Here's how the part is built. I have some questions about the finished solid (model axes, mm). A direction names the side the tool comes from. Round coordinates to 2 decimals unless told otherwise and drop trailing zeros. Loops run counter-clockwise (first coordinate to the right, second up) from the corner with the lowest first, then second, coordinate; pieces in that order, holes last. Notation, with made-up numbers: (75.25, -14.5) -> (128.25, -14.5) arc R14 ccw to (128.25, 10.5) -> close; hole circle Ø11 at (5, 22.25). An arc over 180 degrees is marked (long way). One line per item, written item: value. Start each with the question number.
```python
from build123d import *

# Parameters (mm, degrees)
CROQUIS1_W              = 20
CROQUIS1_H              = 20
SALIENTE_EXTRUIR1_DEPTH = 75
CROQUIS2_R              = 2.5
CORTAR_EXTRUIR2_DEPTH   = 10


with BuildPart() as part:
    # Croquis1 → Saliente-Extruir1 (new, symmetric)
    with BuildSketch(Plane.XY):
        Rectangle(CROQUIS1_W, CROQUIS1_H)
    extrude(amount=SALIENTE_EXTRUIR1_DEPTH, both=True)

    # Croquis2 → Cortar-Extruir2 (cut)
    with BuildSketch(Plane(origin=(0, 0, -75), x_dir=(-1, 0, 0), z_dir=(0, 0, -1))):
        Circle(CROQUIS2_R)
    extrude(amount=-CORTAR_EXTRUIR2_DEPTH, mode=Mode.SUBTRACT)


solid = part.part
```
Q1. If I drill on line 1 along Y through (x, z) = (0, -71); line 2 along Z through (x, y) = (1.25, -0.75), over which ranges is the centre line in solid material (lowest first)?
Q2. I want a section at A-A on y = 0. Please give me the cut outline in (x, z).
Q3. Will this pin go through, and if not, where does the flat tip stop? P1, Ø2.5, axis at x = 0, y = 0.5, coming from the -Z side.
Q4. Which directions (+Z, -Z, +X, -X, +Y, -Y) give clear straight access to the entire face, cutting with the end or side of a thin tool? Please do faces 1 (the cylindrical face through (0.54, -2.44, -70.07)), 2 (the flat face through (-10, 0, 1)).
Q5. If we mould it in two halves opening along Y, with no side actions, what happens to faces 3 (the flat face through (0, 10, 1)), 4 (the flat face through (0, 0, -65)), 5 (the flat face through (-2, -2, -75))? For each: released by +Y, released by -Y, zero draft, split by the parting line, or undercut.
Answers below:
1. line 1: y = -10 to -2.5, 2.5 to 10
1. line 2: z = -65 to 75
2. outline: (-10, -75) -> (-2.5, -75) -> (-2.5, -65) -> (2.5, -65) -> (2.5, -75) -> (10, -75) -> (10, 75) -> (-10, 75) -> close
3. P1: stops at z = -65
4. face 1: -Z
4. face 2: +Z, -Z, -X, +Y, -Y
5. face 3: released by +Y
5. face 4: undercut
5. face 5: zero draft
